The figure shows three views and two pictorial views of one solid part (mm, origin at its lowest corner). Answer the questions. A direction names the side the tool comes from. Coordinates: 2 decimals unless noted, no trailing zeros. Order: outer loops, then holes, each group sorted by start corner. A loop starts at its lowest first (then second) coordinate and runs counter-clockwise, first axis right, second up.
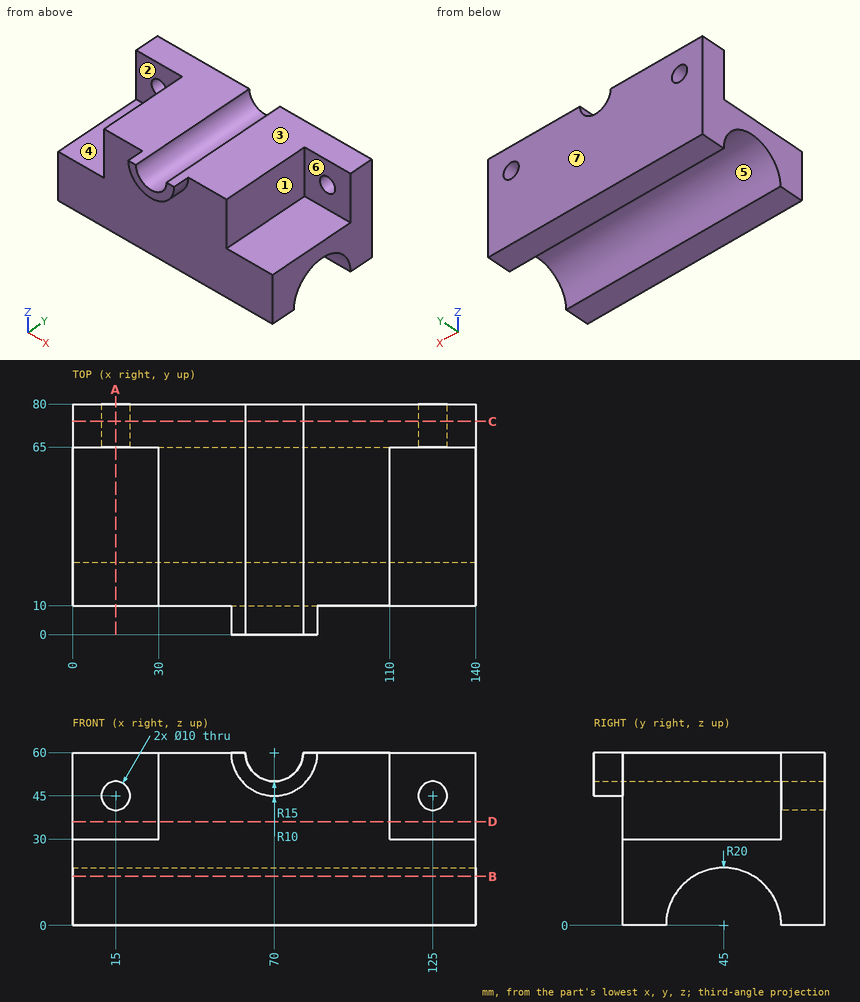
1) A cutting plane is placed at C-C, the plane y = 74. Write down the section's boundary in (x, z), plus the area to 3 significant figures.
2) A cutting plane is placed at B-B, the plane z = 17. Write down the section's boundary in (x, y).
3) Each of these flat-tipped pins is pushed along its axis until it touches: P1, Ø10, axis at x = 45.5, z = 21.5, coming from the -Y side; P2, Ø9, axis at y = 44, z = 47, coming from the -X side; P3, Ø9, axis at x = 15, z = 45, coming from the -Y side; P4, Ø15, axis at x = 14.5, z = 48, coming from the -Y side. Where does it stop, or does it pass through?
4) A cutting plane is placed at A-A, the plane x = 15. Write down the section's boundary in (y, z).
5) The mould has two halves that part along Y. Classify the marked faces 4, 5, 6 and 7: released by +Y, released by -Y, zero draft, split by the parting line, or undercut.
6) A cutting plane is placed at D-D, the plane z = 36. Write down the section's boundary in (x, y), plus the area to 3 significant figures.
7) For the marked faces 1, 2 and 3, determine the directions among +Z, -Z, +X, -X, +Y, -Y from which every point of the face is accessible in a straight line to the end or side of a thin tool.
8) Straight lines are drawn through the part: probe 1 along Z at (x, y) = (15, 74.5); probe 2 along Y at (x, z) = (68, 39); probe 3 along Z at (x, y) = (14.5, 18). For each, find the intervals that lie inside material, in ascending order.
Working result:
1. outline: (0, 0) - (140, 0) - (140, 60) - (80, 60) arc R10 cw to (60, 60) - (0, 60) - close; hole circle Ø10 at (15, 45); hole circle Ø10 at (125, 45)
1. area: 8,090 mm2
2. outline: (0, 10) - (140, 10) - (140, 34.46) - (0, 34.46) - close; (0, 55.54) - (140, 55.54) - (140, 80) - (0, 80) - close
3. P1: stops at y = 10
3. P2: stops at x = 30
3. P3: passes through
3. P4: stops at y = 65
4. outline: (10, 0) - (25, 0) arc R20 cw to (65, 0) - (80, 0) - (80, 40) - (65, 40) - (65, 30) - (10, 30) - close; (65, 50) - (80, 50) - (80, 60) - (65, 60) - close
5. face 4: zero draft
5. face 5: undercut
5. face 6: released by -Y
5. face 7: released by +Y
6. outline: (0, 65) - (30, 65) - (30, 10) - (110, 10) - (110, 65) - (140, 65) - (140, 80) - (0, 80) - close
6. area: 6,500 mm2
7. face 1: +Z, +X, -Y
7. face 2: +Z, -X, -Y
7. face 3: +Z, +X, -X, +Y, -Y
8. probe 1: z = 0 to 40, 50 to 60
8. probe 2: y = 10 to 80
8. probe 3: z = 0 to 30
